Job drawing, mm, ordinate dimensions from the low corner. One solid piece. A direction names the side the tool comes from. Give positions to 0.01 mm unless a question says otherwise; leave off trailing zeros. Loops run counter-clockwise (first coordinate to the right, second up) from the corner with the lowest first, then second, coordinate; pieces in that order, holes last. Notation, with made-up numbers: M 8,11 L 44,11 A15 ccw 44,34 Z; hole C -4,54 d3. An arc over 180 degrees is marked long. One line per question, with ' | ' between items.
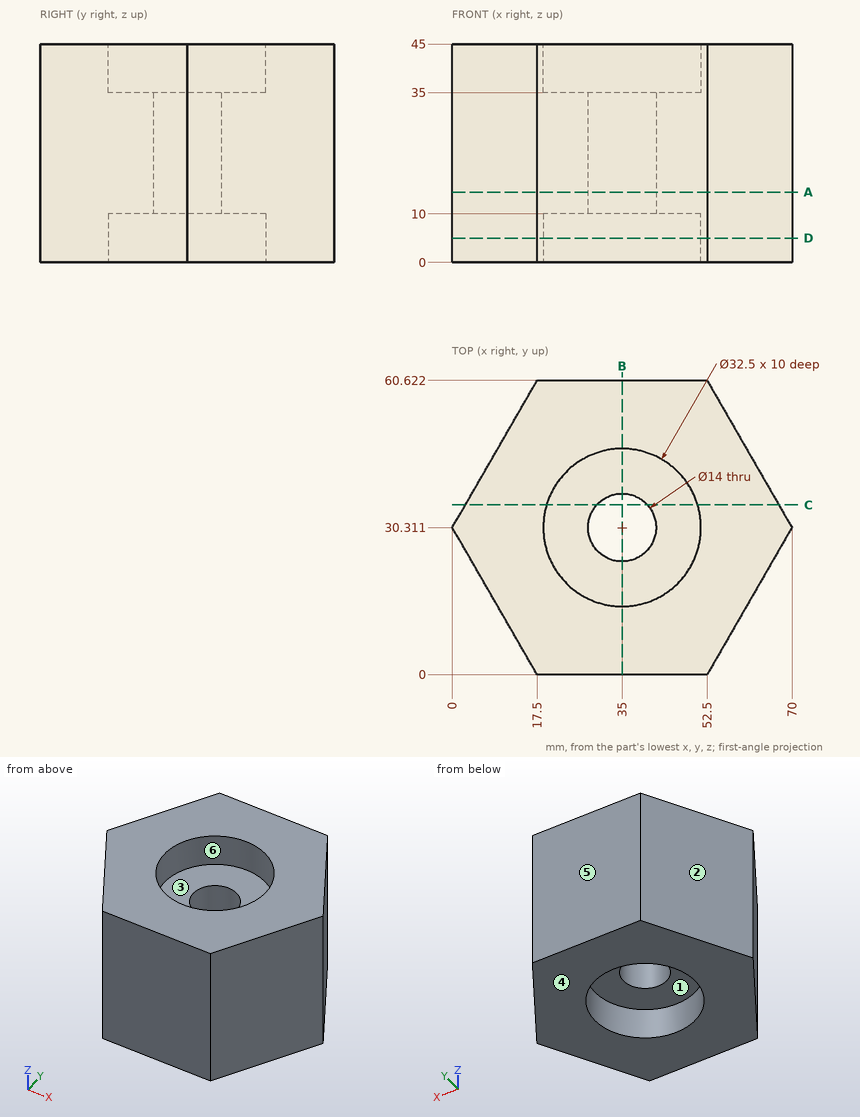
Item 1: Saw through at C-C on y = 35. Give the cut face in (x, z), and give its area (3 significant figures).
Conclusion:
outline: M 2.71,0 L 19.44,0 L 19.44,10 L 29.8,10 L 29.8,35 L 19.44,35 L 19.44,45 L 2.71,45 Z; M 40.2,10 L 50.56,10 L 50.56,0 L 67.29,0 L 67.29,45 L 50.56,45 L 50.56,35 L 40.2,35 Z | area: 2,020 mm²
Item 2: Drop flat-ended pins along their axis: P1, Ø5, axis at y = 12.5, z = 10, coming from the +X side; P2, Ø5, axis at y = 49, z = 18.5, coming from the +X side; P3, Ø19.5, axis at x = 35, y = 30.31, coming from the +Z side. Give the stop position or say it passes through.
Conclusion:
P1: x = 61.16 | P2: x = 60.65 | P3: z = 35
Item 3: Mould opens along Y. For the marked faces 4, 5 and 6 say: pulls with the +Y half, pulls with the -Y half, needs draft (parallel to the pull), parting line crosses it, or undercut.
Conclusion:
face 4: needs draft | face 5: pulls with the +Y half | face 6: undercut
Item 4: Drill centre lines: line 1 along Y through (x, z) = (35, 2.5); line 2 along Y through (x, z) = (35, 15.25); line 3 along X through (y, z) = (32, 29) (1 decimal). Where is each one in solid material? Low to high. Write a range as [from, to].
Conclusion:
line 1: [0, 14.06], [46.56, 60.62] | line 2: [0, 23.31], [37.31, 60.62] | line 3: [1, 28.2], [41.8, 69]
Item 5: Saw through at A-A on z = 14.5. Give the cut face in (x, y).
Conclusion:
outline: M 0,30.31 L 17.5,0 L 52.5,0 L 70,30.31 L 52.5,60.62 L 17.5,60.62 Z; hole C 35,30.31 d14
Item 6: Saw through at B-B on x = 35. Give the cut face in (y, z), and give its area (3 significant figures).
Conclusion:
outline: M 0,0 L 14.06,0 L 14.06,10 L 23.31,10 L 23.31,35 L 14.06,35 L 14.06,45 L 0,45 Z; M 37.31,10 L 46.56,10 L 46.56,0 L 60.62,0 L 60.62,45 L 46.56,45 L 46.56,35 L 37.31,35 Z | area: 1,730 mm²
Item 7: Saw through at D-D on z = 5. Give the cut face in (x, y), and give its area (3 significant figures).
Conclusion:
outline: M 0,30.31 L 17.5,0 L 52.5,0 L 70,30.31 L 52.5,60.62 L 17.5,60.62 Z; hole C 35,30.31 d32.5 | area: 2,350 mm²
Item 8: 3-axis set-ups, long thin cutter, end or side, ignore diameter. For the marked faces 1, 2 and 3: which of +Z, -Z, +X, -X, +Y, -Y reach the whole face in a straight line?
Conclusion:
face 1: -Z | face 2: +Z, -Z, -X, +Y | face 3: +Z
